```python
from build123d import *

# Parameters (mm, degrees)
CYLINDER005_R            = 1.6
CYLINDER005_DEPTH        = 30
PAD002_DEPTH             = 4
CLONE007_PLACEMENT_ANGLE = 59.5063808355
CLONE181_PLACEMENT_ANGLE = 1.91645e-05


with BuildPart() as finger_drill_master:
    # Cylinder005 → Cylinder005 (new body)
    with BuildSketch(Plane.XY.offset(-8)):
        Circle(CYLINDER005_R)
    extrude(amount=CYLINDER005_DEPTH)


with BuildPart() as clone006:
    # Clone006 base: copy of finger-drill-master
    add(finger_drill_master.part)


with BuildPart() as clone006_1:
    # Clone006 placement: moved
    add(clone006.part.moved(Location((40, 0, 0))))


with BuildPart() as fusion012:
    # Clone005 base: copy of finger-drill-master
    add(finger_drill_master.part)

    # Fusion012: union Clone006
    add(clone006_1.part)


with BuildPart() as clone_of_left_link:
    # Sketch002 → Pad002 (new body)
    with BuildSketch(Plane.XY):
        with BuildLine():
            ThreePointArc((0, 3.7), (-3.7, 0), (0, -3.7))
            Line((0, -3.7), (40, -3.7))
            ThreePointArc((40, -3.7), (43.7, 0), (40, 3.7))
            Line((0, 3.7), (40, 3.7))
        make_face()
    extrude(amount=PAD002_DEPTH)

    # Cut001: cut Fusion012
    add(fusion012.part, mode=Mode.SUBTRACT)


with BuildPart() as clone_of_left_link_1:
    # Clone007 placement: moved
    add(clone_of_left_link.part.moved(Location((187.1034801236, 214.4662976869, 4.3))).rotate(Axis((187.1034801236, 214.4662976869, 4.3), (0, 0, 1)), CLONE007_PLACEMENT_ANGLE))


with BuildPart() as clone_of_left_link_2:
    # Clone181 placement: moved
    add(clone_of_left_link_1.part.moved(Location((-14.0004083881, -699.0003602699, 7.3))).rotate(Axis((-14.0004083881, -699.0003602699, 7.3), (0, 0, 1)), CLONE181_PLACEMENT_ANGLE))


solid = clone_of_left_link_2.part
```
The model under review builds one solid part; all positions refer to its coordinate system, in mm. Round coordinates to 2 decimals unless told otherwise and drop trailing zeros. Write each loop counter-clockwise with the first axis right and the second up, starting at its lowest first coordinate (ties: lowest second). Pieces come first, ordered by that corner, then holes. Notation, with made-up numbers: (64, 15.25) - (73, 15.25) arc R24 ccw to (73, 28.25) - close; hole circle Ø7 at (-16, 48.5). An arc over 180 degrees is marked (long way). Answer as CSV lines item,"result". Start each with the question number.
(1) We need section C-C on y = -449.5. State the section outline as (x, z) points, plus the area to 3 significant figures.
(2) Draft analysis for pull direction X (two halves, no side actions). For faces 1 (the cylindrical face through (192.675, -448.641, 13.572)), 2 (the flat face through (186.298, -469.419, 13.572)), 3 (the cylindrical face through (195.35, -446.92, 13.57)), state which applies: pulls with the +X half, pulls with the -X half, needs draft (parallel to the pull), parting line crosses it, or undercut.
(3) We need section D-D on x = 184. State the section outline as (y, z) points.
(4) We need section B-B on z = 14.55. State the section outline as (x, y) points, plus the area to 3 significant figures.
(5) To check wall thickness, follow line 1 (X direction, y = -483.5, z = 14.2); line 2 (Y direction, x = 192.25, z = 14.7); line 3 (Y direction, x = 172.25, z = 14.6). State the ranges of each line that lie inside material, in increasing order.
(6) For pin 1 Ø3.5 at (x, y) = (173.103, -484.534) entering from -Z; pin 2 Ø1.5 at (x, z) = (179.5, 15) entering from -Y; pin 3 Ø2 at (y, z) = (-463.5, 13.5) entering from -X, all flat-tipped, find the tip position at first contact; note any pin that passes through.
(7) We need section A-A on y = -484. State the section outline as (x, z) points.
Worked answers:
1,outline,"(189.44, 11.6) - (191.9, 11.6) - (191.9, 15.6) - (189.44, 15.6) - close; (194.9, 11.6) - (197.06, 11.6) - (197.06, 15.6) - (194.9, 15.6) - close"
1,area,"18.5 mm²"
2,face 1,"undercut"
2,face 2,"pulls with the +X half"
2,face 3,"parting line crosses it"
3,outline,"(-473.32, 11.6) - (-458.74, 11.6) - (-458.74, 15.6) - (-473.32, 15.6) - close"
4,outline,"(169.91, -482.66) arc R3.7 ccw to (176.29, -486.41) - (196.59, -451.94) arc R3.7 ccw to (190.21, -448.19) - close; hole circle Ø3.2 at (173.1, -484.53); hole circle Ø3.2 at (193.4, -450.07)"
4,area,"323 mm²"
5,line 1,"169.55 to 171.88, 174.32 to 178.01"
5,line 2,"-459.31 to -451.18, -448.95 to -446.55"
5,line 3,"-488.13 to -485.89, -483.18 to -478.69"
6,pin 1,"z = 11.6"
6,pin 2,"y = -482.24"
6,pin 3,"x = 180.61"
7,outline,"(169.44, 11.6) - (171.59, 11.6) - (171.59, 15.6) - (169.44, 15.6) - close; (174.61, 11.6) - (177.71, 11.6) - (177.71, 15.6) - (174.61, 15.6) - close"
